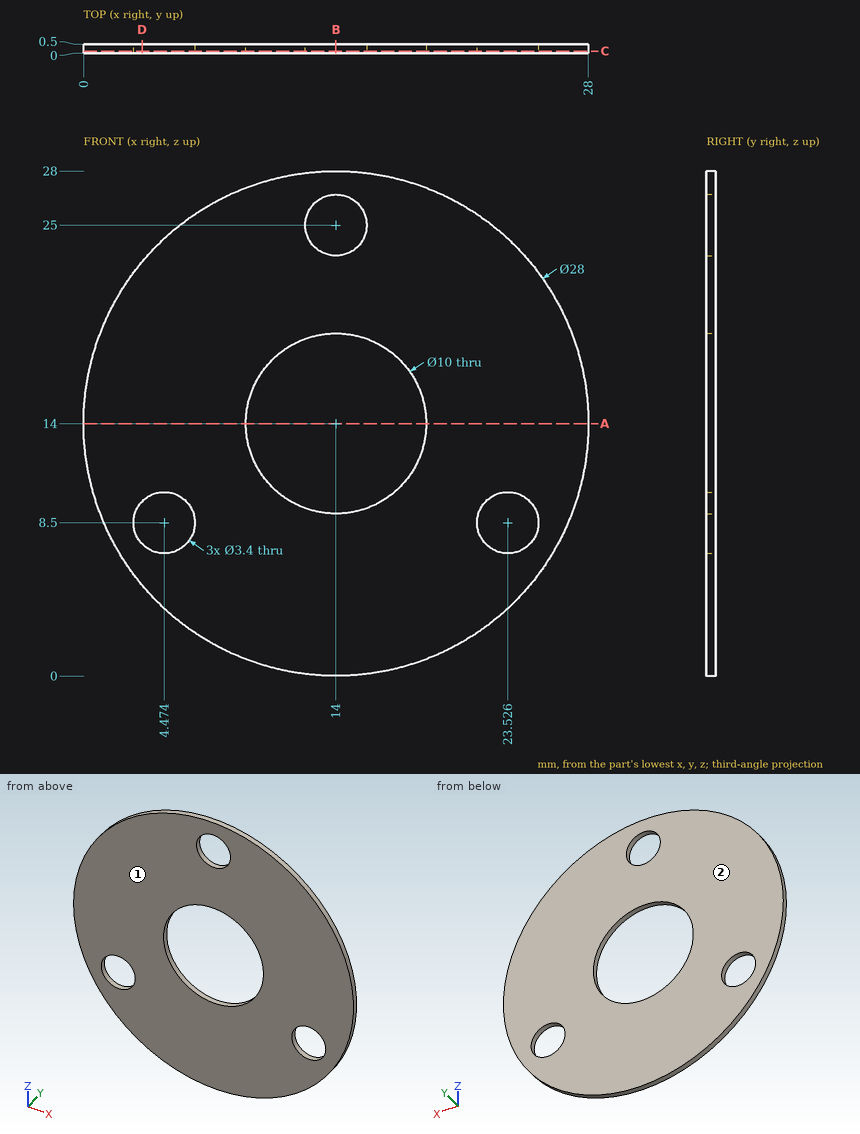
Could you check a few things on this drawing? It's one solid part, dimensions in mm from its lowest x, y, z. Give positions to 0.01 mm unless a question says otherwise; leave off trailing zeros. Order: outer loops, then holes, each group sorted by start corner. A loop starts at its lowest first (then second) coordinate and runs counter-clockwise, first axis right, second up. Notation, with made-up numbers: (43.5, 85.25) -> (61.5, 85.25) arc R21 ccw to (61.5, 114.25) -> close; hole circle Ø2 at (30.25, -6.75). An arc over 180 degrees is marked (long way). Answer in a Markdown table with one row per item. Add a question column.
Item 1: I'm going to push a flat-ended pin straight in: P1, Ø2.5, axis at x = 23.53, z = 8.5, coming from the -Y side. Where does the tip first touch, or does it pass through?
Item 2: Imagine slicing it at D-D (x = 3.25). List the corners of the cut face in (y, z) for me.
Item 3: Imagine slicing it at B-B (x = 14). List the corners of the cut face in (y, z) for me.
Item 4: We'd pull the mould along Y, two halves only. Please class the marked faces 1 and 2: pulls with the +Y half, pulls with the -Y half, needs draft (parallel to the pull), parting line crosses it, or undercut.
Item 5: Please list where these lines run through material, in increasing order: probe 1 along X at (y, z) = (0.3, 8.5) (1 decimal); probe 2 along Z at (x, y) = (14.5, 0.3) (1 decimal); probe 3 along Z at (x, y) = (15.25, 0.05) (1 decimal).
Item 6: Imagine slicing it at C-C (y = 0.1). List the corners of the cut face in (x, z) for me.
Item 7: Imagine slicing it at A-A (z = 14). List the corners of the cut face in (x, y) for me.
Result:
| question | item | result |
|---|---|---|
| 1 | P1 | through |
| 2 | outline | (0, 5.03) -> (0.5, 5.03) -> (0.5, 7.32) -> (0, 7.32) -> close; (0, 9.68) -> (0.5, 9.68) -> (0.5, 22.97) -> (0, 22.97) -> close |
| 3 | outline | (0, 0) -> (0.5, 0) -> (0.5, 9) -> (0, 9) -> close; (0, 19) -> (0.5, 19) -> (0.5, 23.3) -> (0, 23.3) -> close; (0, 26.7) -> (0.5, 26.7) -> (0.5, 28) -> (0, 28) -> close |
| 4 | face 1 | pulls with the -Y half |
| 4 | face 2 | pulls with the +Y half |
| 5 | probe 1 | 1.1 to 2.8, 6.2 to 21.8, 25.2 to 26.9 |
| 5 | probe 2 | 0 to 9, 19 to 23.4, 26.6 to 28 |
| 5 | probe 3 | 0.1 to 9.2, 18.8 to 23.8, 26.2 to 27.9 |
| 6 | outline | circle Ø28 at (14, 14); hole circle Ø3.4 at (4.47, 8.5); hole circle Ø10 at (14, 14); hole circle Ø3.4 at (14, 25); hole circle Ø3.4 at (23.53, 8.5) |
| 7 | outline | (0, 0) -> (9, 0) -> (9, 0.5) -> (0, 0.5) -> close; (19, 0) -> (28, 0) -> (28, 0.5) -> (19, 0.5) -> close |
